from build123d import *

# Parameters (mm, degrees)
EXTRUDE_1_DEPTH     = 1.5
SKETCH_2_R          = 1
EXTRUDE_2_DEPTH     = 2.25
SKETCH_3_R          = 0.85
CUT_EXTRUDE_1_DEPTH = 3


with BuildPart() as part:
    # Эскиз1 → Бобышка-Вытянуть1 (new body)
    with BuildSketch(Plane.XY):
        with BuildLine():
            Line((-1, 0), (-1.5, 0))
            ThreePointArc((-1.5, 0), (-2.207106781, 0.292893219), (-2.5, 1))
            Line((-2.5, 1), (-2.5, 24))
            Line((-2.5, 24), (0, 24))
            Line((0, 24), (0, 1))
            ThreePointArc((0, 1), (-0.292893219, 0.292893219), (-1, 0))
        make_face()
    extrude(amount=EXTRUDE_1_DEPTH)

    # Эскиз2 → Бобышка-Вытянуть2 (add)
    with BuildSketch(Plane.XY.offset(1.5)):
        with Locations((-1.25, 6)):
            Circle(SKETCH_2_R)
    extrude(amount=EXTRUDE_2_DEPTH)

    # Эскиз3 → Вырез-Вытянуть1 (cut)
    with BuildSketch(Plane(origin=(0, 24, 0), x_dir=(1, 0, 0), z_dir=(0, 1, 0))):
        with Locations((-1.25, -0.75)):
            Circle(SKETCH_3_R)
    extrude(amount=-CUT_EXTRUDE_1_DEPTH, mode=Mode.SUBTRACT)


solid = part.part
Geometry: final body of the model. Coordinates: model frame, mm. A direction names the side the tool comes from. Round coordinates to 2 decimals unless told otherwise and drop trailing zeros. Loops run counter-clockwise (first coordinate to the right, second up) from the corner with the lowest first, then second, coordinate; pieces in that order, holes last. Notation, with made-up numbers: M 13.5,-5.5 L 24.5,-5.5 A31 cw 24.5,26.5 Z; hole C -28.75,16 d4. An arc over 180 degrees is marked long. Put each result on its own line as item: value. Start each with the question number.
(1) Material intervals for line 1 along Z through (x, y) = (-0.3, 14.5); line 2 along Y through (x, z) = (-1.25, 3.3); line 3 along X through (y, z) = (21.75, 0.9), sorted ascending. Write a range as [from, to].
(2) Contact query for flat-ended pins moving along their axis: pin 1 Ø0.8 at (x, y) = (-1, 15) entering from +Z; pin 2 Ø1 at (x, y) = (-1.5, 5) entering from +Z; pin 3 Ø0.8 at (x, z) = (-1, 0.5) entering from +Y. Output: stop coordinate, or through.
(3) Section query C-C (z = 1). Return loops of the section in (x, y), then the cut area to 3 significant figures.
(4) Section query B-B (y = 6). Return loops of the section in (x, z).
(5) Set-up query: faces 5 (the face through (-0.2, 24, 0.7)), 6 (the face through (-1.38, 6.99, 2.61)), 7 (the face through (-2.1, 22.5, 0.7)). Return all of +Z, -Z, +X, -X, +Y, -Y with unobstructed straight access to the full face (end or side cutting, diameter ignored); none if empty.
(6) Section query D-D (y = 13.5). Return loops of the section in (x, z).
(7) Section query A-A (x = -1.25). Return loops of the section in (y, z).
(8) Draft query along X for faces 1 (the face through (-1, 12, 1.5)), 2 (the face through (-0.4, 22.5, 0.8)), 3 (the face through (-1, 21, 1)), 4 (the face through (0, 13, 1)). Return one class per face: +X half, -X half, draft (parallel to the pull), parting line (faces both ways), or undercut.
Findings below:
1. line 1: z = [0, 1.5]
1. line 2: y = [5, 7]
1. line 3: x = [-2.5, -2.09], [-0.41, 0]
2. pin 1: stops at z = 1.5
2. pin 2: stops at z = 3.75
2. pin 3: stops at y = 21
3. outline: M -2.5,1 A1 ccw -1.5,0 L -1,0 A1 ccw 0,1 L 0,24 L -0.44,24 L -0.44,21 L -2.06,21 L -2.06,24 L -2.5,24 Z
3. area: 54.7 mm2
4. outline: M -2.5,0 L 0,0 L 0,1.5 L -0.25,1.5 L -0.25,3.75 L -2.25,3.75 L -2.25,1.5 L -2.5,1.5 Z
5. face 5: +Z, -Z, +X, -X, +Y
5. face 6: +Z
5. face 7: +Y
6. outline: M -2.5,0 L 0,0 L 0,1.5 L -2.5,1.5 Z
7. outline: M 0,0 L 21,0 L 21,1.5 L 7,1.5 L 7,3.75 L 5,3.75 L 5,1.5 L 0,1.5 Z
8. face 1: draft
8. face 2: undercut
8. face 3: undercut
8. face 4: +X half
